from build123d import *

# Parameters (mm, degrees)
SKETCH1_R            = 18
SKETCH1_R_2          = 15
BOSS_EXTRUDE1_DEPTH  = 80
BOSS_EXTRUDE2_DEPTH  = 5
BOSS_EXTRUDE4_DEPTH  = 10
SKETCH3_R            = 25
SKETCH3_R_2          = 20
SKETCH3_R_3          = 18
SKETCH3_R_4          = 13.000000000000002
BOSS_EXTRUDE6_DEPTH  = 5
SKETCH15_W           = 29.000000000000004
SKETCH15_H           = 9
BOSS_EXTRUDE13_DEPTH = 20
SKETCH16_R           = 5.5
CUT_EXTRUDE3_DEPTH   = 89.85521931771932
FILLET1_R            = 2


with BuildPart() as part:
    # Sketch1 → Boss-Extrude1 (new body)
    with BuildSketch(Plane(origin=(0, 0, 0), x_dir=(1, 0, 0), z_dir=(0, 1, 0))):
        with Locations(Location((0, 0, 0), (0, 0, 270))):
            Circle(SKETCH1_R)
        with Locations(Location((0, 0, 0), (0, 0, 270))):
            Circle(SKETCH1_R_2, mode=Mode.SUBTRACT)
    extrude(amount=BOSS_EXTRUDE1_DEPTH)

    # Sketch1_3 → Boss-Extrude2 (add)
    with BuildSketch(Plane(origin=(0, 0, 0), x_dir=(1, 0, 0), z_dir=(0, 1, 0))):
        with BuildLine():
            ThreePointArc((14.488887394336022, 3.8822856765378235), (10.606601717798192, 10.606601717798233), (3.8822856765377662, 14.488887394336036))
            Line((3.882285676537766, 14.488887394336036), (3.3646475863327305, 12.557035741757899))
            ThreePointArc((3.3646475863327314, 12.557035741757902), (9.192388155425101, 9.192388155425139), (12.557035741757888, 3.364647586332781))
            Line((12.557035741757888, 3.3646475863327807), (14.488887394336023, 3.882285676537824))
        make_face()
        with BuildLine():
            ThreePointArc((15, 0), (14.871672920607155, 1.9578928833007803), (14.488887394336022, 3.8822856765378235))
            Line((14.488887394336023, 3.882285676537824), (12.557035741757888, 3.3646475863327807))
            ThreePointArc((12.557035741757888, 3.364647586332781), (12.888783197859539, 1.6968404988606767), (13.000000000000004, 0))
            ThreePointArc((13.000000000000004, -3.18e-15), (12.888783197859537, -1.696840498860684), (12.557035741757888, -3.364647586332781))
            Line((12.557035741757888, -3.364647586332778), (14.488887394336023, -3.882285676537821))
            ThreePointArc((14.488887394336022, -3.8822856765378235), (14.871672920607153, -1.9578928833007887), (15, -3.67e-15))
        make_face()
        with BuildLine():
            ThreePointArc((3.8822856765377662, -14.488887394336036), (10.606601717798192, -10.606601717798233), (14.488887394336022, -3.8822856765378235))
            Line((14.488887394336023, -3.882285676537821), (12.557035741757888, -3.364647586332778))
            ThreePointArc((12.557035741757888, -3.364647586332781), (9.192388155425101, -9.192388155425139), (3.3646475863327314, -12.557035741757902))
            Line((3.3646475863327305, -12.5570357417579), (3.882285676537766, -14.488887394336036))
        make_face()
        with BuildLine():
            ThreePointArc((-3.882285676537771, -14.488887394336034), (-2.76e-15, -15), (3.8822856765377662, -14.488887394336036))
            Line((3.882285676537766, -14.488887394336036), (3.3646475863327305, -12.5570357417579))
            ThreePointArc((3.3646475863327314, -12.557035741757902), (-2.39e-15, -13.000000000000004), (-3.364647586332736, -12.5570357417579))
            Line((-3.3646475863327305, -12.557035741757899), (-3.8822856765377654, -14.488887394336034))
        make_face()
        with BuildLine():
            Line((-12.557035741757886, -3.3646475863327807), (-14.488887394336022, -3.882285676537824))
            ThreePointArc((-14.488887394336022, -3.8822856765378244), (-10.606601717798195, -10.606601717798231), (-3.882285676537771, -14.488887394336034))
            Line((-3.8822856765377654, -14.488887394336034), (-3.3646475863327305, -12.557035741757899))
            ThreePointArc((-3.364647586332736, -12.5570357417579), (-9.192388155425105, -9.192388155425135), (-12.557035741757888, -3.364647586332782))
        make_face()
        with BuildLine():
            Line((-12.557035741757888, 3.3646475863327785), (-14.488887394336022, 3.882285676537821))
            ThreePointArc((-14.488887394336022, 3.8822856765378218), (-15, 1.84e-15), (-14.488887394336022, -3.8822856765378244))
            Line((-14.488887394336022, -3.882285676537824), (-12.557035741757886, -3.3646475863327807))
            ThreePointArc((-12.557035741757888, -3.364647586332782), (-13.000000000000004, 1.59e-15), (-12.557035741757888, 3.36464758633278))
        make_face()
        with BuildLine():
            Line((-3.3646475863327305, 12.5570357417579), (-3.882285676537766, 14.488887394336036))
            ThreePointArc((-3.8822856765377676, 14.488887394336036), (-10.606601717798194, 10.606601717798231), (-14.488887394336022, 3.8822856765378218))
            Line((-14.488887394336022, 3.882285676537821), (-12.557035741757888, 3.3646475863327785))
            ThreePointArc((-12.557035741757888, 3.36464758633278), (-9.192388155425103, 9.192388155425137), (-3.36464758633273, 12.557035741757902))
        make_face()
        with BuildLine():
            Line((3.3646475863327305, 12.557035741757899), (3.882285676537766, 14.488887394336036))
            ThreePointArc((3.8822856765377662, 14.488887394336036), (9.2e-16, 15), (-3.8822856765377676, 14.488887394336036))
            Line((-3.882285676537766, 14.488887394336036), (-3.3646475863327305, 12.5570357417579))
            ThreePointArc((-3.36464758633273, 12.557035741757902), (8e-16, 13.000000000000004), (3.3646475863327314, 12.557035741757902))
        make_face()
    extrude(amount=BOSS_EXTRUDE2_DEPTH)

    # Sketch1_4 → Boss-Extrude4 (add)
    with BuildSketch(Plane(origin=(0, 0, 0), x_dir=(1, 0, 0), z_dir=(0, 1, 0))):
        with BuildLine():
            Line((-12.557035741757888, 3.3646475863327785), (-14.488887394336022, 3.882285676537821))
            ThreePointArc((-14.488887394336022, 3.8822856765378218), (-15, 1.84e-15), (-14.488887394336022, -3.8822856765378244))
            Line((-14.488887394336022, -3.882285676537824), (-12.557035741757886, -3.3646475863327807))
            ThreePointArc((-12.557035741757888, -3.364647586332782), (-13.000000000000004, 1.59e-15), (-12.557035741757888, 3.36464758633278))
        make_face()
        with BuildLine():
            Line((3.3646475863327305, 12.557035741757899), (3.882285676537766, 14.488887394336036))
            ThreePointArc((3.8822856765377662, 14.488887394336036), (9.2e-16, 15), (-3.8822856765377676, 14.488887394336036))
            Line((-3.882285676537766, 14.488887394336036), (-3.3646475863327305, 12.5570357417579))
            ThreePointArc((-3.36464758633273, 12.557035741757902), (8e-16, 13.000000000000004), (3.3646475863327314, 12.557035741757902))
        make_face()
        with BuildLine():
            ThreePointArc((-3.882285676537771, -14.488887394336034), (-2.76e-15, -15), (3.8822856765377662, -14.488887394336036))
            Line((3.882285676537766, -14.488887394336036), (3.3646475863327305, -12.5570357417579))
            ThreePointArc((3.3646475863327314, -12.557035741757902), (-2.39e-15, -13.000000000000004), (-3.364647586332736, -12.5570357417579))
            Line((-3.3646475863327305, -12.557035741757899), (-3.8822856765377654, -14.488887394336034))
        make_face()
        with BuildLine():
            ThreePointArc((15, 0), (14.871672920607155, 1.9578928833007803), (14.488887394336022, 3.8822856765378235))
            Line((14.488887394336023, 3.882285676537824), (12.557035741757888, 3.3646475863327807))
            ThreePointArc((12.557035741757888, 3.364647586332781), (12.888783197859539, 1.6968404988606767), (13.000000000000004, 0))
            ThreePointArc((13.000000000000004, -3.18e-15), (12.888783197859537, -1.696840498860684), (12.557035741757888, -3.364647586332781))
            Line((12.557035741757888, -3.364647586332778), (14.488887394336023, -3.882285676537821))
            ThreePointArc((14.488887394336022, -3.8822856765378235), (14.871672920607153, -1.9578928833007887), (15, -3.67e-15))
        make_face()
    extrude(amount=BOSS_EXTRUDE4_DEPTH)

    # Sketch3 → Boss-Extrude6 (add)
    # profile 1 of 3: a face of its own
    with BuildSketch(Plane.XZ):
        with Locations(Location((0, 0, 0), (0, 0, 270))):
            Circle(SKETCH3_R)
        Circle(SKETCH3_R_2, mode=Mode.SUBTRACT)
    # profile 2 of 3: a face of its own
    with BuildSketch(Plane.XZ):
        Circle(SKETCH3_R_2)
        with Locations(Location((0, 0, 0), (0, 0, 270))):
            Circle(SKETCH3_R_3, mode=Mode.SUBTRACT)
    # profile 3 of 3: a face of its own
    with BuildSketch(Plane.XZ):
        Circle(SKETCH3_R_4)
    extrude(amount=-BOSS_EXTRUDE6_DEPTH)

    # Sketch15 → Boss-Extrude13 (add)
    with BuildSketch(Plane.XZ):
        Rectangle(SKETCH15_W, SKETCH15_H)
    extrude(amount=BOSS_EXTRUDE13_DEPTH)

    # Sketch16 → Cut-Extrude3 (cut, through all)
    with BuildSketch(Plane.XY.offset(4.500000000000001)):
        with Locations((0, -12)):
            Circle(SKETCH16_R)
    extrude(amount=-CUT_EXTRUDE3_DEPTH, mode=Mode.SUBTRACT)

    # Fillet1
    fillet1_edges = [part.edges().sort_by_distance(p)[0] for p in [
        (-5.08e-15, 5, -18),
        (14.5, 0, 0),
        (14.5, -10, -4.5),
        (0, 0, 4.500000000000001),
        (14.5, -10, 4.500000000000001),
        (-14.5, 0, 8.9e-16),
        (-14.5, -10, 4.500000000000001),
        (0, 0, -4.5),
        (-14.5, -10, -4.5),
        (14.5, -20, 0),
        (0, -20, 4.500000000000001),
        (-14.5, -20, 8.9e-16),
        (0, -20, -4.5),
    ]]
    fillet(fillet1_edges, radius=FILLET1_R)


solid = part.part
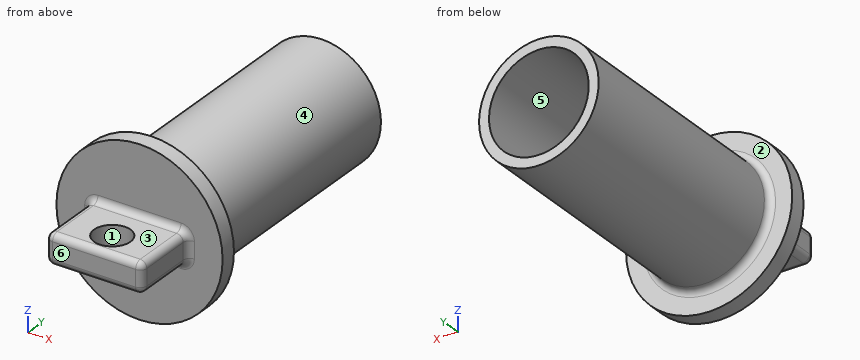
Design review of the part built by this model. Coordinates are the model's own, in mm. Face numbers are marked on the shaded views. A direction names the side the tool comes from. Round coordinates to 2 decimals unless told otherwise and drop trailing zeros. Write each loop counter-clockwise with the first axis right and the second up, starting at its lowest first coordinate (ties: lowest second). Pieces come first, ordered by that corner, then holes.
Item 1: For the marked faces 1, 2 and 3, list the 3-axis set-ups (+Z, -Z, +X, -X, +Y, -Y) from which the entire face can be reached by the end or side of a thin tool; tool diameter is ignored.
Item 2: Wall thickness on L1, parallel to X at y = 35, z = 0; L2, parallel to Y at x = -9, z = -1.5: over which ranges is each line inside the solid? List them lowest first.
Item 3: Draft analysis for pull direction X (two halves, no side actions). For the marked faces 4, 5 and 6, state which applies: released by +X, released by -X, zero draft, split by the parting line, or undercut.
Item 4: For pin 1 Ø8 at (x, y) = (5, -10.5) entering from -Z; pin 2 Ø4 at (y, z) = (-9, 0) entering from +X; pin 3 Ø6 at (x, y) = (12, 53.5) entering from -Z; pin 4 Ø10 at (x, z) = (-14, 1) entering from -Y, all flat-tipped, find the tip position at first contact; note any pin that passes through.
Item 5: Consider section B-B on z = 0. Give the boundary of the cut face in (x, y).
Item 6: Consider section D-D on y = 24. Give the boundary of the cut face in (x, z).
Item 7: Consider section C-C on y = -12. Give the boundary of the cut face in (x, z).
Check values:
1. face 1: +Z, -Z
1. face 2: +Y
1. face 3: +Z, +X, -X, -Y
2. L1: x = -18 to -15, 15 to 18
2. L2: y = -20 to 5
3. face 4: split by the parting line
3. face 5: undercut
3. face 6: zero draft
4. pin 1: stops at z = -4.5
4. pin 2: stops at x = 14.5
4. pin 3: stops at z = -15.59
4. pin 4: stops at y = -20
5. outline: (-25, 0) - (-16.5, 0) arc R2 cw to (-14.5, -2) - (-14.5, -18) arc R2 ccw to (-12.5, -20) - (12.5, -20) arc R2 ccw to (14.5, -18) - (14.5, -2) arc R2 cw to (16.5, 0) - (25, 0) - (25, 5) - (20, 5) arc R2 cw to (18, 7) - (18, 80) - (15, 80) - (15, 10) - (13, 10) - (13, 5) - (-13, 5) - (-13, 10) - (-15, 10) - (-15, 80) - (-18, 80) - (-18, 7) arc R2 cw to (-20, 5) - (-25, 5) - close; hole circle Ø11 at (0, -12)
6. outline: circle Ø36 at (0, 0); hole circle Ø30 at (0, 0)
7. outline: (-14.5, -2.5) arc R2 ccw to (-12.5, -4.5) - (-5.5, -4.5) - (-5.5, 4.5) - (-12.5, 4.5) arc R2 ccw to (-14.5, 2.5) - close; (5.5, -4.5) - (12.5, -4.5) arc R2 ccw to (14.5, -2.5) - (14.5, 2.5) arc R2 ccw to (12.5, 4.5) - (5.5, 4.5) - close
